```python
from build123d import *
from build123d.topology import SkipClean

# Parameters (mm, degrees)
ESTRUSIONE_ESTRUSIONE1_DEPTH      = 6
ESTRUSIONE_ESTRUSIONE2_DEPTH      = 5
ESTRUSIONE_ESTRUSIONE3_DEPTH      = 21
ESTRUSIONE_ESTRUSIONE3_DEPTH_BACK = 6


with BuildPart() as part:
    # Schizzo1 → Estrusione-Estrusione1 (new, symmetric)
    with SkipClean():  # the faces are left unmerged after this step: merging them gives an invalid solid
        with BuildSketch(Plane(origin=(0, 0, 0), x_dir=(1, 0, 0), z_dir=(0, 1, 0))):
            with BuildLine():
                ThreePointArc((-83.089397902, 0), (-78.089397902, 5), (-73.089397902, 0))
                Line((-73.089397902, 0), (-68.089397902, 0))
                ThreePointArc((-68.089397902, 0), (-71.356394609, 7.393691004), (-79.022731235, 9.956349175))
                ThreePointArc((-79.022731235, 9.956349175), (-85.483088906, 6.733003292), (-88.089397902, 0))
                Line((-88.089397902, 0), (-83.089397902, 0))
            make_face()
            with BuildLine():
                Line((-68.089397902, 0), (-73.089397902, 0))
                ThreePointArc((-73.089397902, 0), (-78.089397902, -5), (-83.089397902, 0))
                Line((-83.089397902, 0), (-88.089397902, 0))
                ThreePointArc((-88.089397902, 0), (-85.483088906, -6.733003292), (-79.022731235, -9.956349175))
                ThreePointArc((-79.022731235, -9.956349175), (-71.356394609, -7.393691004), (-68.089397902, 0))
            make_face()
        extrude(amount=ESTRUSIONE_ESTRUSIONE1_DEPTH, both=True)

    # Schizzo1_3 → Estrusione-Estrusione2 (add, symmetric)
    with SkipClean():  # the faces are left unmerged after this step: merging them gives an invalid solid
        with BuildSketch(Plane(origin=(0, 0, 0), x_dir=(1, 0, 0), z_dir=(0, 1, 0))):
            with BuildLine():
                ThreePointArc((-79.022731235, 9.956349175), (-71.356394609, 7.393691004), (-68.089397902, 0))
                Line((-68.089397902, 0), (-20.089397902, 0))
                ThreePointArc((-20.089397902, 0), (-15.658672609, 11.446105597), (-4.676064568, 16.925793597))
                Line((-4.676064568, 16.925793597), (-79.022731235, 9.956349175))
            make_face()
            with BuildLine():
                Line((-20.089397902, 0), (-68.089397902, 0))
                ThreePointArc((-68.089397902, 0), (-71.356394609, -7.393691004), (-79.022731235, -9.956349175))
                Line((-79.022731235, -9.956349175), (-4.676064568, -16.925793597))
                ThreePointArc((-4.676064568, -16.925793597), (-15.658672609, -11.446105597), (-20.089397902, 0))
            make_face()
        extrude(amount=ESTRUSIONE_ESTRUSIONE2_DEPTH, both=True)

    # Schizzo1_4 → Estrusione-Estrusione3 (add, two sides: drawn at the far end of the back side and taken through both)
    with SkipClean():  # the faces are left unmerged after this step: merging them gives an invalid solid
        with BuildSketch(Plane(origin=(0, 0, 0), x_dir=(1, 0, 0), z_dir=(0, 1, 0)).offset(-ESTRUSIONE_ESTRUSIONE3_DEPTH_BACK)):
            with BuildLine():
                ThreePointArc((-4.676064568, 16.925793597), (-15.658672609, 11.446105597), (-20.089397902, 0))
                Line((-20.089397902, 0), (-15.628789916, 0))
                Line((-15.628789916, 0), (-15.628789916, 3))
                Line((-15.628789916, 3), (-12.628789916, 3))
                ThreePointArc((-12.628789916, 3), (-1.571820909, 9.884177258), (6.910602098, 0))
                Line((6.910602098, 0), (13.910602098, 0))
                ThreePointArc((13.910602098, 0), (8.356707695, 12.569274707), (-4.676064568, 16.925793597))
            make_face()
            with BuildLine():
                Line((-15.628789916, 0), (-20.089397902, 0))
                ThreePointArc((-20.089397902, 0), (-15.658672609, -11.446105597), (-4.676064568, -16.925793597))
                ThreePointArc((-4.676064568, -16.925793597), (8.356707695, -12.569274707), (13.910602098, 0))
                Line((13.910602098, 0), (6.910602098, 0))
                ThreePointArc((6.910602098, 0), (-1.571820909, -9.884177258), (-12.628789916, -3))
                Line((-12.628789916, -3), (-15.628789916, -3))
                Line((-15.628789916, -3), (-15.628789916, 0))
            make_face()
        extrude(amount=ESTRUSIONE_ESTRUSIONE3_DEPTH + ESTRUSIONE_ESTRUSIONE3_DEPTH_BACK)


solid = part.part
```
Design review of the part built by this model. Coordinates are the model's own, in mm. A direction names the side the tool comes from. Give positions to 0.01 mm unless a question says otherwise; leave off trailing zeros. Order: outer loops, then holes, each group sorted by start corner. A loop starts at its lowest first (then second) coordinate and runs counter-clockwise, first axis right, second up. Notation, with made-up numbers: (71, 53.25) -> (129, 53.25) arc R32 ccw to (129, 84.25) -> close; hole circle Ø1 at (13, 16.5). An arc over 180 degrees is marked (long way). Write item = value, one per line. Start each with the question number.
(1) We need section D-D on z = 13.5. Write out the cut boundary in (x, y), plus the area to 3 significant figures.
(2) To check wall thickness, follow line 1 along X through (y, z) = (7, 0.5); line 2 along Y through (x, z) = (-58.5, -0.5); line 3 along X through (y, z) = (1.25, -2). State the ranges of each line that lie inside material, in increasing order.
(3) For pin 1 (8 mm diameter, centred on x = -36.5, y = 5, fed in from +Z); pin 2 (17 mm diameter, centred on x = -34, z = 0, fed in from -Y); pin 3 (6 mm diameter, centred on x = -60, z = 9.5, fed in from +Y); pin 4 (12 mm diameter, centred on x = -38, y = 12, fed in from -Z), all flat-tipped, find the tip position at first contact; note any pin that passes through.
(4) For faces 5 (the face through (-14, 7, 3)), 6 (the face through (4.2, -6, 7.3)), list the 3-axis set-ups (+Z, -Z, +X, -X, +Y, -Y) from which the entire face can be reached by the end or side of a thin tool; tool diameter is ignored.
(5) Mouldability with a two-part tool opening along Z and no side actions: class faces 1 (the face through (-15.629, 7, 0)), 2 (the face through (-42.37, 0.07, 13.392)), 3 (the face through (-41.33, 0.07, -13.49)), 4 (the face through (-42, -5, 0)) as +Z half, -Z half, draft (parallel to the pull), parting line (faces both ways), or undercut.
(6) We need section B-B on y = -2. Write out the cut boundary in (x, z).
(7) We need section A-A on y = 15.75. Write out the cut boundary in (x, z).
(8) We need section C-C on x = -78. Write out the cut boundary in (y, z), plus the area to 3 significant figures.
Numbers:
q1.outline = (-41.22, -5) -> (-13.42, -5) -> (-13.42, -6) -> (7.24, -6) -> (7.24, 21) -> (-13.42, 21) -> (-13.42, 5) -> (-41.22, 5) -> close
q1.area = 836 mm^2
q2.line_1 = -20.08 to -15.63, 6.9 to 13.9
q2.line_2 = -5 to 5
q2.line_3 = -87.89 to -82.67, -73.51 to -15.63, 6.71 to 13.79
q3.pin_1 = 14.32
q3.pin_2 = -5
q3.pin_3 = 5
q3.pin_4 = through
q4.face_5 = +Y, -Y
q4.face_6 = +Z, -Z, +X, -X, -Y
q5.face_1 = undercut
q5.face_2 = +Z half
q5.face_3 = -Z half
q5.face_4 = draft
q6.outline = (-79.02, -9.96) -> (-4.68, -16.93) arc R17 ccw (long way) to (-4.68, 16.93) -> (-79.02, 9.96) arc R10 ccw to start; hole circle Ø10 at (-78.09, 0); hole (-15.63, -3) -> (-12.63, -3) arc R10 ccw (long way) to (-12.63, 3) -> (-15.63, 3) -> close
q7.outline = circle Ø34 at (-3.09, 0); hole (-15.63, -3) -> (-12.63, -3) arc R10 ccw (long way) to (-12.63, 3) -> (-15.63, 3) -> close
q8.outline = (-6, -10) -> (-5, -10) -> (-5, -10.05) -> (5, -10.05) -> (5, -10) -> (6, -10) -> (6, -5) -> (-6, -5) -> close; (-6, 5) -> (6, 5) -> (6, 10) -> (5, 10) -> (5, 10.05) -> (-5, 10.05) -> (-5, 10) -> (-6, 10) -> close
q8.area = 121 mm^2
